Solid Edge part; units mm, degrees
sketch "Sketch1" plane through (0, 0, 0) normal (0, 0, 1) x (1, 0, 0)
  line L0 (0, -7.2579) -> (56, -7.2579)
  line L1 (56, -7.2579) -> (56, 17.2421)
  line L2 (56, 17.2421) -> (0, 17.2421)
  line L3 (0, 17.2421) -> (0, -7.2579)
extrude "Protrusion1" add sketch "Sketch1" along normal blind 23.9
hole "Hole_1" at (52.5, 12.7421, 23.9) direction (0, 0, -1) diameter 3.3 end through all
hole "Hole1" at (3.5, 12.7421, 23.9) direction (0, 0, -1) diameter 3.3 end through all
sketch "Sketch2" plane through (28, 4.9921, 23.9) normal (0, 0, 1) x (1, 0, 0)
  line L0 (-28, 12.25) -> (28, 12.25)
  line L1 (28, 12.25) -> (28, 11.25)
  line L2 (28, 11.25) -> (-28, 11.25)
  line L3 (-28, 11.25) -> (-28, 12.25)
extrude "Cutout1" cut sketch "Sketch2" against normal through all
properties material "Aluminum, 6061-T6"
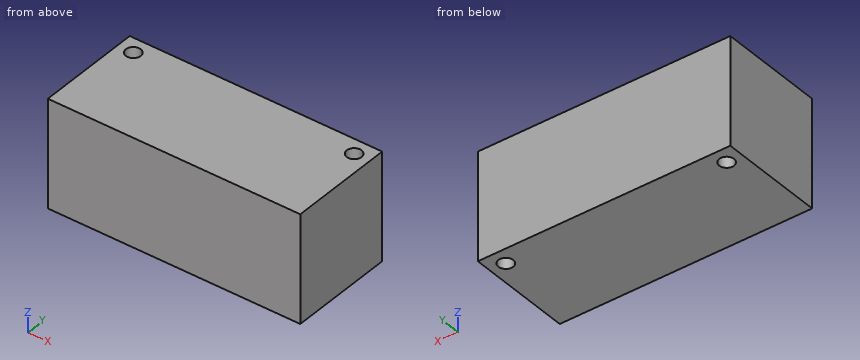
Check sheet for the modelled part. Datum: model origin and axes. Units: mm. Coordinates: 2 decimals unless noted, no trailing zeros. Write each loop counter-clockwise with the first axis right and the second up, starting at its lowest first coordinate (ties: lowest second). Pieces come first, ordered by that corner, then holes. Notation, with made-up numbers: M 19.25,-17.75 L 47.25,-17.75 A17 ccw 47.25,-7.75 Z; hole C -33.5,33 d2. An arc over 180 degrees is marked long. Use one line per item in the form item = value.
Item 1: Sectioned sample at A-A, the plane x = 3.5. Record the cut outline in (y, z).
Answer below:
outline = M -7.26,0 L 11.09,0 L 11.09,23.9 L -7.26,23.9 Z; M 14.39,0 L 16.24,0 L 16.24,23.9 L 14.39,23.9 Z
Item 2: Material ranges on L1, parallel to Y at x = 3.5, z = 5.5; L2, parallel to X at y = 13, z = 12.5; L3, parallel to X at y = 14, z = 21, recorded low to high. Write a range as from..to.
Answer below:
L1 = -7.26..11.09, 14.39..16.24
L2 = 0..1.87, 5.13..50.87, 54.13..56
L3 = 0..2.43, 4.57..51.43, 53.57..56
Item 3: Sectioned sample at B-B, the plane y = 13.5. Record the cut outline in (x, z), and give its area (3 significant figures).
Answer below:
outline = M 0,0 L 2.03,0 L 2.03,23.9 L 0,23.9 Z; M 4.97,0 L 51.03,0 L 51.03,23.9 L 4.97,23.9 Z; M 53.97,0 L 56,0 L 56,23.9 L 53.97,23.9 Z
area = 1,200 mm^2
